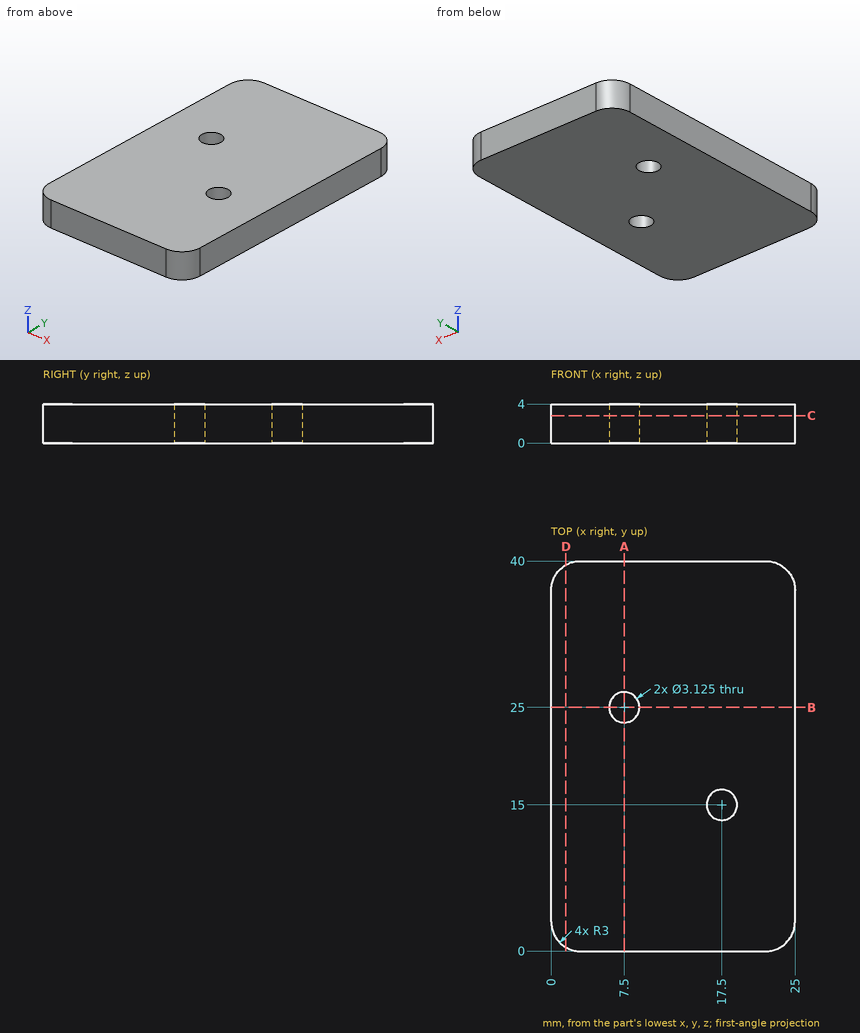
Can you work these out from the drawing? Everything is in mm from the part's minimum corner. Round coordinates to 2 decimals unless told otherwise and drop trailing zeros. Loops run counter-clockwise (first coordinate to the right, second up) from the corner with the lowest first, then second, coordinate; pieces in that order, holes last. Notation, with made-up numbers: (83, 37.25) - (106, 37.25) arc R12 cw to (106, 54.25) - close; hole circle Ø6 at (41, -29.5). An arc over 180 degrees is marked (long way). Answer as CSV lines item,"result".
1. I want a section at B-B on y = 25. List the corners of the cut face in (x, z) for me.
Filled in:
outline,"(0, 0) - (5.94, 0) - (5.94, 4) - (0, 4) - close; (9.06, 0) - (25, 0) - (25, 4) - (9.06, 4) - close"
2. I want a section at D-D on x = 1.5. List the corners of the cut face in (y, z) for me, then the cut area to 3 significant figures.
Filled in:
outline,"(0.4, 0) - (39.6, 0) - (39.6, 4) - (0.4, 4) - close"
area,"157 mm^2"
3. I want a section at A-A on x = 7.5. List the corners of the cut face in (y, z) for me, then the cut area to 4 significant figures.
Filled in:
outline,"(0, 0) - (23.44, 0) - (23.44, 4) - (0, 4) - close; (26.56, 0) - (40, 0) - (40, 4) - (26.56, 4) - close"
area,"147.5 mm^2"
4. I want a section at C-C on z = 2.8. List the corners of the cut face in (x, y) for me (1 decimal), then the cut area to 3 significant figures.
Filled in:
outline,"(0, 3) arc R3 ccw to (3, 0) - (22, 0) arc R3 ccw to (25, 3) - (25, 37) arc R3 ccw to (22, 40) - (3, 40) arc R3 ccw to (0, 37) - close; hole circle Ø3.1 at (7.5, 25); hole circle Ø3.1 at (17.5, 15)"
area,"977 mm^2"
5. Please list where these lines run through material, in increasing order: line 1 along Y through (x, z) = (7.5, 1.2); line 2 along Y through (x, z) = (17.5, 1.65); line 3 along Y through (x, z) = (1.75, 1.85). Write a range as [from, to].
Filled in:
line 1,"y = [0, 23.44], [26.56, 40]"
line 2,"y = [0, 13.44], [16.56, 40]"
line 3,"y = [0.27, 39.73]"
